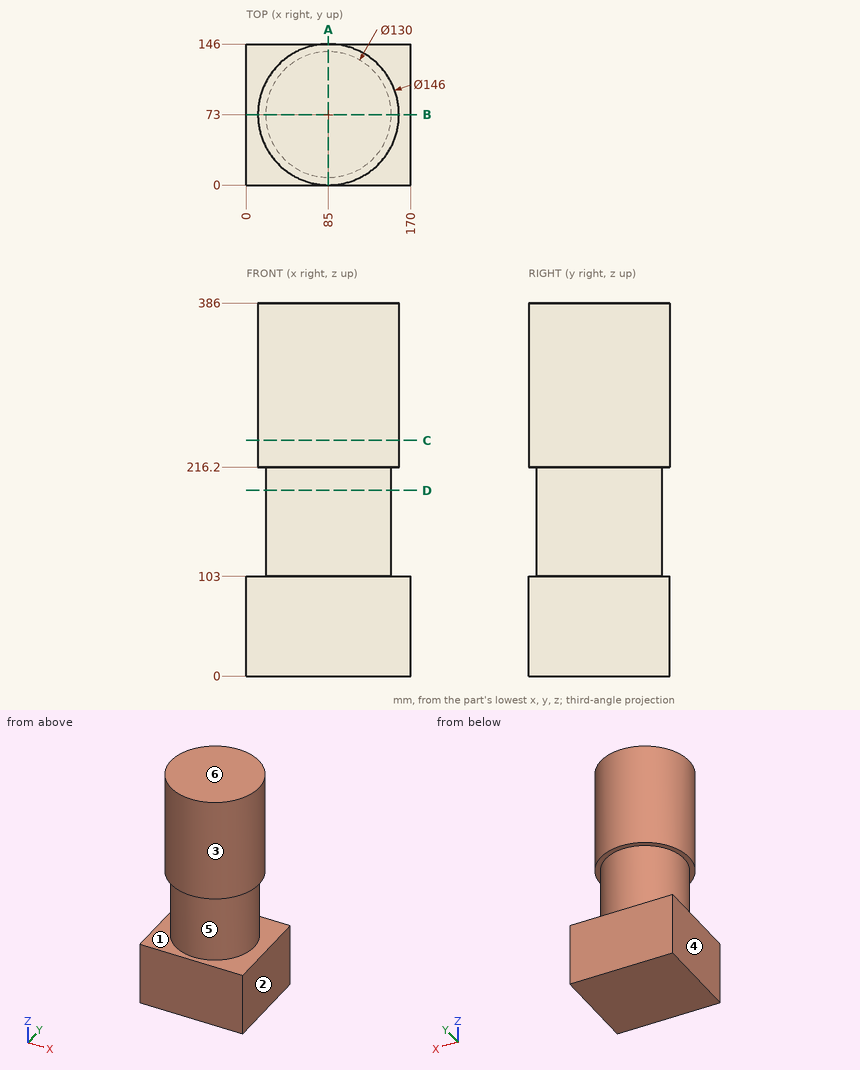
Input: dimensioned drawing with shaded views. Units: mm. Origin: part minimum x, y, z. A direction names the side the tool comes from. Give positions to 0.01 mm unless a question says otherwise; leave off trailing zeros. Write each loop counter-clockwise with the first axis right and the second up, starting at its lowest first coordinate (ties: lowest second). Pieces come first, ordered by that corner, then holes.
1. Section query C-C, the plane z = 244. Return loops of the section in (x, y).
2. Section query D-D, the plane z = 192. Return loops of the section in (x, y).
3. Section query A-A, the plane x = 85. Return loops of the section in (y, z), then the cut area to 3 significant figures.
4. Draft query along Z for the marked faces 4, 5 and 6. Return one class per face: released by +Z, released by -Z, zero draft, split by the parting line, or undercut.
5. Section query B-B, the plane y = 73. Return loops of the section in (x, z).
6. Line query: probe 1 along Z at (x, y) = (143.5, 8); probe 2 along Y at (x, z) = (81.5, 222); probe 3 along X at (y, z) = (50, 370.5). Output: solid intervals per line, ascending.
7. Pin query (flat end, axial travel): P1, Ø12, axis at x = 109, z = 263.5, coming from the +Y side; P2, Ø3, axis at y = 43, z = 209.5, coming from the -X side; P3, Ø6, axis at x = 113.5, z = 337, coming from the +Y side. Return the tip coordinate at first contact, or that it passes through.
8. Reachability of the marked faces 1, 2 and 3 from +Z, -Z, +X, -X, +Y, -Y: full face, straight path, thin tool, end or side. Return the list, or none.
Computed:
1. outline: circle Ø146 at (85, 73)
2. outline: circle Ø130 at (85, 73)
3. outline: (0, 0) - (146, 0) - (146, 103) - (138, 103) - (138, 216.2) - (146, 216.2) - (146, 386) - (0, 386) - (0, 216.2) - (8, 216.2) - (8, 103) - (0, 103) - close
3. area: 54,500 mm2
4. face 4: zero draft
4. face 5: undercut
4. face 6: released by +Z
5. outline: (0, 0) - (170, 0) - (170, 103) - (150, 103) - (150, 216.2) - (158, 216.2) - (158, 386) - (12, 386) - (12, 216.2) - (20, 216.2) - (20, 103) - (0, 103) - close
6. probe 1: z = 0 to 103
6. probe 2: y = 0.08 to 145.92
6. probe 3: x = 15.72 to 154.28
7. P1: stops at y = 143.75
7. P2: stops at x = 26.58
7. P3: stops at y = 141.4
8. face 1: none
8. face 2: +Z, -Z, +X, +Y, -Y
8. face 3: +Z
